Check sheet for the modelled part. Datum: model origin and axes. Units: mm. Coordinates: 2 decimals unless noted, no trailing zeros. Write each loop counter-clockwise with the first axis right and the second up, starting at its lowest first coordinate (ties: lowest second). Pieces come first, ordered by that corner, then holes. Notation, with made-up numbers: M 71.5,62.25 L 75.5,62.25 A19 ccw 75.5,99.25 Z; hole C 29,-7 d4. An arc over 180 degrees is marked long. Answer as CSV lines item,"result". Start each with the question number.
Q1. Thickness scan on line 1 along X through (y, z) = (2, 2.6); line 2 along X through (y, z) = (6, 2.7); line 3 along X through (y, z) = (7.5, 0.8). Record the ranges inside material, lowest first. Write a range as from..to.
Q2. Sectioned sample at C-C, the plane z = 0.6. Record the cut outline in (x, y), then the cut area to 3 significant figures.
Q3. Sectioned sample at B-B, the plane y = 0. Record the cut outline in (x, z).
Q4. Sectioned sample at A-A, the plane x = 0. Record the cut outline in (y, z), then the cut area to 3 significant figures.
Q5. Sectioned sample at D-D, the plane z = 1.8. Record the cut outline in (x, y).
Q6. Depth check by flat-ended pin: pin 1 Ø0.8 at (x, y) = (-1.5, -0.5) entering from +Z; pin 2 Ø1 at (y, z) = (2, 1.5) entering from -X. Enter the tip coordinate at first touch or a pass-through.
Solid Edge part; units mm, degrees
sketch "Sketch1" plane through (0, 0, 0) normal (0, -1, 0) x (1, 0, 0)
  line L0 (0, 0) -> (9, 0)
  line L1 (9, 0) -> (7.5, 3)
  line L2 (7.5, 3) -> (0, 3)
  dimension "D1" = 9
  dimension "D2" = 7.5
revolve "RevolvedProtrusion1" add sketch "Sketch1" angle 360 about axis through (0, 0, 3) along (0, 0, -1)
sketch "Sketch2" plane through (0, 0, 3) normal (0, 0, 1) x (1, 0, 0)
  line L0 (-2, -4) -> (-1, -4)
  line L1 (-1, -4) -> (-1, 4)
  line L2 (-1, 4) -> (-2, 4)
  line L3 (-2, 4) -> (-2, -4)
  line L4 (2, -4) -> (1, -4)
  line L5 (1, -4) -> (1, 4)
  line L6 (1, 4) -> (2, 4)
  line L7 (2, 4) -> (2, -4)
  dimension "D1" = 1
  dimension "D2" = 2
extrude "Cutout1" cut sketch "Sketch2" against normal blind 0.5
fillet "main_rounds" radius 0.25 10 edges at (1.5, 4, 3) (2, 0, 3) (-1.5, 4, 3) (-2, 0, 3) (-1, 0, 3) (-1.5, -4, 3) (1, 0, 3) (1.5, -4, 3) (-9, 0, 0) (-7.5, 0, 3)
properties material "Polyethylene, low density"
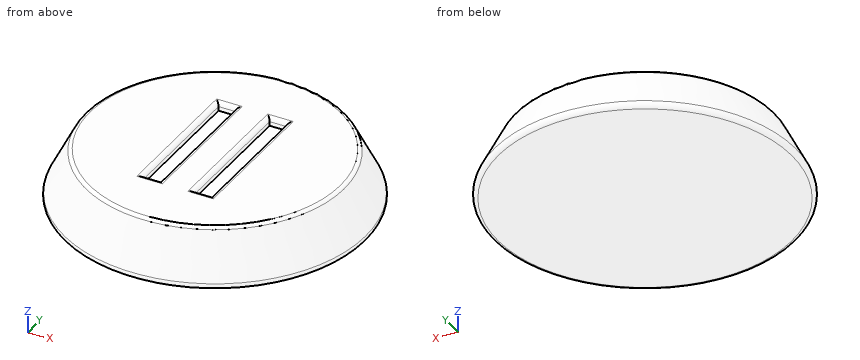
Output:
1,line 1,"x = -7.44..-2, -1..1, 2..7.44"
1,line 2,"x = -4.75..4.75"
1,line 3,"x = -4.21..4.21"
2,outline,"C 0,0 d17.4"
2,area,"238 mm^2"
3,outline,"M -8.82,0.36 A0.25 ccw -8.6,0 L 8.6,0 A0.25 ccw 8.82,0.36 L 7.57,2.86 A0.25 ccw 7.35,3 L 2.25,3 A0.25 ccw 2,2.75 L 2,2.5 L 1,2.5 L 1,2.75 A0.25 ccw 0.75,3 L -0.75,3 A0.25 ccw -1,2.75 L -1,2.5 L -2,2.5 L -2,2.75 A0.25 ccw -2.25,3 L -7.35,3 A0.25 ccw -7.57,2.86 Z"
4,outline,"M -8.82,0.36 A0.25 ccw -8.6,0 L 8.6,0 A0.25 ccw 8.82,0.36 L 7.57,2.86 A0.25 ccw 7.35,3 L -7.35,3 A0.25 ccw -7.57,2.86 Z"
4,area,"49.4 mm^2"
5,outline,"C 0,0 d16.2"
6,pin 1,"stops at z = 2.5"
6,pin 2,"stops at x = -8.29"
